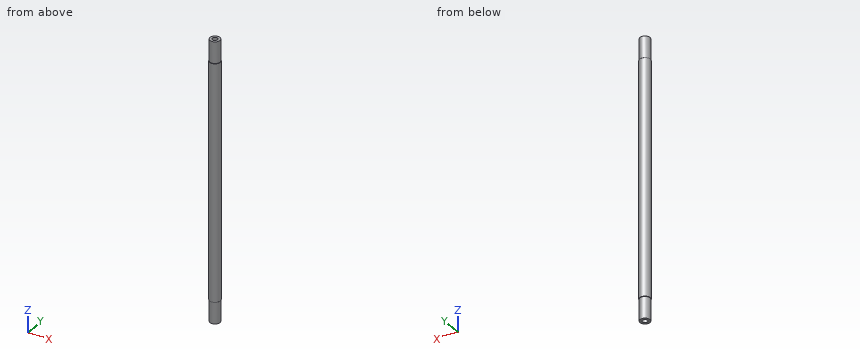
```python
from build123d import *

# Parameters (mm, degrees)
SKETCH_1_R          = 40
SKETCH_1_R_2        = 20
EXTRUDE_1_DEPTH     = 2082
SKETCH_2_R          = 40
SKETCH_2_R_2        = 37.5
CUT_EXTRUDE_1_DEPTH = 160
CUT_EXTRUDE_START   = -160
SKETCH_3_R          = 40
SKETCH_3_R_2        = 37.5
CUT_EXTRUDE_2_DEPTH = 160
CHAMFER_1_SIZE      = 1


with BuildPart() as part:
    # 草图1 → 凸台-拉伸1 (new body)
    with BuildSketch(Plane.XY):
        Circle(SKETCH_1_R)
        Circle(SKETCH_1_R_2, mode=Mode.SUBTRACT)
    extrude(amount=EXTRUDE_1_DEPTH)

    # 草图2 → 切除-拉伸1 (cut)
    with BuildSketch(Plane(origin=(0, 0, 0), x_dir=(-1, 0, 0), z_dir=(0, 0, -1))):
        Circle(SKETCH_2_R)
        Circle(SKETCH_2_R_2, mode=Mode.SUBTRACT)
    extrude(amount=-CUT_EXTRUDE_1_DEPTH, mode=Mode.SUBTRACT)

    # 草图3 → 切除-拉伸2 (cut)
    with BuildSketch(Plane.XY.offset(2082).offset(CUT_EXTRUDE_START)):
        with Locations(Location((0, 0, 0), (0, 0, 180))):
            Circle(SKETCH_3_R)
        with Locations(Location((0, 0, 0), (0, 0, 180))):
            Circle(SKETCH_3_R_2, mode=Mode.SUBTRACT)
    extrude(amount=CUT_EXTRUDE_2_DEPTH, mode=Mode.SUBTRACT)

    # 倒角1
    chamfer_1_edges = [part.edges().sort_by_distance(p)[0] for p in [
        (-40, 0, 160),
        (-40, 0, 1922),
    ]]
    chamfer(chamfer_1_edges, length=CHAMFER_1_SIZE)


solid = part.part
```
Input: part model. Units: mm. Frame: model coordinates. Give positions to 0.01 mm unless a question says otherwise; leave off trailing zeros. Write each loop counter-clockwise with the first axis right and the second up, starting at its lowest first coordinate (ties: lowest second). Pieces come first, ordered by that corner, then holes. Notation, with made-up numbers: (-25, -12.5) - (-6, -12.5) arc R23 ccw to (-6, -2.5) - close; hole circle Ø4 at (78.5, 26.25). An arc over 180 degrees is marked (long way). Write item = value, one per line. Start each with the question number.
1) Cut plane C-C (z = 1641). Return loops of the section in (x, y), and give its area (3 significant figures).
2) Material intervals for L1, parallel to X at y = 1, z = 428.5; L2, parallel to Y at x = 0, z = 582; L3, parallel to X at y = -1.5, z = 1030.5, sorted ascending. Write a range as [from, to].
3) Pin query (flat end, axial travel): pin 1 (1.5 mm diameter, centred on y = 5, z = 887.5, fed in from -X); pin 2 (12 mm diameter, centred on x = 7, z = 754.5, fed in from -Y); pin 3 (4 mm diameter, centred on x = -9.5, z = 638.5, fed in from +Y). Return the tip coordinate at first contact, or that it passes through.
4) Cut plane A-A (x = 0). Return loops of the section in (y, z), and give its area (3 significant figures).
Answers follow:
q1.outline = circle Ø80 at (0, 0); hole circle Ø40 at (0, 0)
q1.area = 3,770 mm^2
q2.L1 = [-39.99, -19.97], [19.97, 39.99]
q2.L2 = [-40, -20], [20, 40]
q2.L3 = [-39.97, -19.94], [19.94, 39.97]
q3.pin_1 = -39.77
q3.pin_2 = -39.99
q3.pin_3 = 39.29
q4.outline = (-40, 161) - (-39, 160) - (-37.5, 160) - (-37.5, 0) - (-20, 0) - (-20, 2082) - (-37.5, 2082) - (-37.5, 1922) - (-39, 1922) - (-40, 1921) - close; (20, 0) - (37.5, 0) - (37.5, 160) - (39, 160) - (40, 161) - (40, 1921) - (39, 1922) - (37.5, 1922) - (37.5, 2082) - (20, 2082) - close
q4.area = 81,700 mm^2
